from build123d import *

# Parameters (mm, degrees)
F1_DEPTH       = 4
F3_D           = 5.5
F3_CSINK_D     = 11.2
F3_CSINK_ANGLE = 90


with BuildPart() as f1:
    # F0 (on Front) → F1 (new body)
    with BuildSketch(Plane.XZ):
        with BuildLine():
            ThreePointArc((-14, 0), (-11.3639610307, -6.3639610307), (-5, -9))
            Line((-5, -9), (5, -9))
            ThreePointArc((5, -9), (11.3639610307, -6.3639610307), (14, 0))
            ThreePointArc((14, 0), (11.3639610307, 6.3639610307), (5, 9))
            Line((5, 9), (-5, 9))
            ThreePointArc((-5, 9), (-11.3639610307, 6.3639610307), (-14, 0))
        make_face()
    extrude(amount=F1_DEPTH)

    # F3 (through all)
    with Locations(Plane.XZ.offset(4)):
        with Locations((0, 0)):
            CounterSinkHole(F3_D / 2, F3_CSINK_D / 2, counter_sink_angle=F3_CSINK_ANGLE)


solid = f1.part
Verification items for the finished model (mm, model axes). Give positions to 0.01 mm unless a question says otherwise; leave off trailing zeros. Write each loop counter-clockwise with the first axis right and the second up, starting at its lowest first coordinate (ties: lowest second). Pieces come first, ordered by that corner, then holes. Notation, with made-up numbers: M 83,-18 L 115,-18 A21 ccw 115,-7 Z; hole C 29.25,6 d10. An arc over 180 degrees is marked long. Put each result on its own line as item: value. Start each with the question number.
1. Section check B-B (x = 0). Record the cut outline in (y, z), and give its area (3 significant figures).
2. Section check A-A (y = -1.5). Record the cut outline in (x, z), and give its area (3 significant figures).
3. Go/stop test with flat-tipped pins: pin 1 Ø1 at (y, z) = (-1.5, 3) entering from -X; pin 2 Ø1 at (y, z) = (-2.5, 4.5) entering from +X. Record where each tip stops, or that it passes through.
4. Scan lines: line 1 along Z through (x, y) = (0, -0.4); line 2 along X through (y, z) = (-0.8, -0.75); line 3 along X through (y, z) = (-2.9, -7.75). Record each from-to range of solid material in increasing order. Write a range as [from, to].
5. Draft check along X on faces 1 (the face through (0, -2, -9)), 2 (the face through (0.596, -0.567, -2.685)). Enter one of: +X half, -X half, draft (parallel to the pull), parting line (faces both ways), or undercut.
6. Section check D-D (z = -6). Record the cut outline in (x, y), and give its area (3 significant figures).
7. Section check C-C (x = 8). Record the cut outline in (y, z).
Answer list:
1. outline: M -4,-9 L 0,-9 L 0,-2.75 L -1.15,-2.75 L -4,-5.6 Z; M -4,5.6 L -1.15,2.75 L 0,2.75 L 0,9 L -4,9 Z
1. area: 41.9 mm2
2. outline: M -5,-9 L 5,-9 A9 ccw 5,9 L -5,9 A9 ccw Z; hole C 0,0 d6.2
2. area: 404 mm2
3. pin 1: x = -13.65
3. pin 2: x = 13.06
4. line 1: [-9, -2.75], [2.75, 9]
4. line 2: [-13.97, -2.65], [2.65, 13.97]
4. line 3: [-9.58, 9.58]
5. face 1: draft
5. face 2: undercut
6. outline: M -11.71,-4 L 11.71,-4 L 11.71,0 L -11.71,0 Z
6. area: 93.7 mm2
7. outline: M -4,-8.49 L 0,-8.49 L 0,8.49 L -4,8.49 Z
